from build123d import *

# Parameters (mm, degrees)
F1_DEPTH    = 924
F2_T1_DEPTH = 1877.7738168108


# Not quite as in the source:
# - a fillet or chamfer that OpenCascade refuses, or shapes differently, is made with other operations: its cross-section is extruded or revolved along the edge and cut away or added


with BuildPart() as f1:
    # F0 (on Right) → F1 (new body, symmetric)
    with BuildSketch(Plane.YZ):
        with BuildLine():
            ThreePointArc((-20.915, -48.8), (-20.3292135624, -50.2142135624), (-18.915, -50.8))
            Line((-18.915, -50.8), (18.915, -50.8))
            ThreePointArc((18.915, -50.8), (20.3292135624, -50.2142135624), (20.915, -48.8))
            Line((20.915, -48.8), (20.915, 48.8))
            ThreePointArc((20.915, 48.8), (20.3292135624, 50.2142135624), (18.915, 50.8))
            Line((18.915, 50.8), (-18.915, 50.8))
            ThreePointArc((-18.915, 50.8), (-20.3292135624, 50.2142135624), (-20.915, 48.8))
            Line((-20.915, 48.8), (-20.915, 44.8355484375))
            Line((-20.915, 44.8355484375), (10.0807787137, 42.1237691829))
            ThreePointArc((10.0807787137, 42.1237691829), (13.3313866841, 40.5207467305), (14.645, 37.1427956924))
            Line((14.645, 37.1427956924), (14.645, -37.1427956924))
            ThreePointArc((14.645, -37.1427956924), (13.3313866841, -40.5207467305), (10.0807787137, -42.1237691829))
            Line((10.0807787137, -42.1237691829), (-20.915, -44.8355484375))
            Line((-20.915, -44.8355484375), (-20.915, -48.8))
        make_face()
    extrude(amount=F1_DEPTH, both=True)

    # F2: fillet of radius 7 on 2 edges, made by hand

    # F2_s2 → F2_t1 (cut)
    with BuildSketch(Plane.YZ.offset(-938.8869084054)):
        with BuildLine():
            ThreePointArc((-20.915, -48.8), (-18.5934823683, -45.7054865005), (-14.9828963102, -44.3165566138))
            Line((-14.9828963102, -44.3165566138), (-14.9950981142, -44.177089356))
            Line((-14.9950981142, -44.177089356), (-20.927201804, -44.6960811798))
            Line((-20.927201804, -44.6960811798), (-21.055, -44.8355484375))
            ThreePointArc((-21.055, -44.8355484375), (-21.055, -46.8177742187), (-21.0458438778, -48.75020161))
            Line((-21.0458438778, -48.75020161), (-20.915, -48.8))
        make_face()
        with BuildLine():
            ThreePointArc((-14.9828963102, 44.3165566138), (-18.5934823683, 45.7054865005), (-20.915, 48.8))
            Line((-20.915, 48.8), (-21.0458438778, 48.75020161))
            ThreePointArc((-21.0458438778, 48.75020161), (-21.055, 46.8177742187), (-21.055, 44.8355484375))
            Line((-21.055, 44.8355484375), (-20.927201804, 44.6960811798))
            Line((-20.927201804, 44.6960811798), (-14.9950981142, 44.177089356))
            Line((-14.9950981142, 44.177089356), (-14.9828963102, 44.3165566138))
        make_face()
    extrude(amount=F2_T1_DEPTH, mode=Mode.SUBTRACT)


solid = f1.part
For this review, take the finished solid that the model builds, in its own axes (mm). A direction names the side the tool comes from. Round coordinates to 2 decimals unless told otherwise and drop trailing zeros. Loops run counter-clockwise (first coordinate to the right, second up) from the corner with the lowest first, then second, coordinate; pieces in that order, holes last. Notation, with made-up numbers: (33, 37.5) - (79, 37.5) arc R21 cw to (79, 44.5) - close; hole circle Ø4 at (3, -15.5). An arc over 180 degrees is marked (long way). Use one line per item in the form item = value.
Item 1: Consider section C-C on z = -1. Write out the cut boundary in (x, y) (3 decimals), then the cut area to 3 significant figures.
Answers:
outline = (-924, 14.645) - (924, 14.645) - (924, 20.915) - (-924, 20.915) - close
area = 11,600 mm^2
Item 2: Consider section A-A on x = -666. Write out the cut boundary in (y, z) (3 decimals).
Answers:
outline = (-20.915, -48.8) arc R2 ccw to (-18.915, -50.8) - (18.915, -50.8) arc R2 ccw to (20.915, -48.8) - (20.915, 48.8) arc R2 ccw to (18.915, 50.8) - (-18.915, 50.8) arc R2 ccw to (-20.915, 48.8) arc R7 ccw to (-14.983, 44.317) - (10.081, 42.124) arc R5 cw to (14.645, 37.143) - (14.645, -37.143) arc R5 cw to (10.081, -42.124) - (-14.983, -44.317) arc R7 ccw to start
Item 3: Clearance check with flat-ended pins moving along their axes: P1, Ø4, axis at x = -621.5, z = -20.5, coming from the -Y side (3 decimals); P2, Ø8, axis at x = -631, z = 37, coming from the -Y side. State where each tip first meets the part, or that it passes through.
Answers:
P1 = 14.645
P2 = 12.83
Item 4: Tool access review of faces 1 (the flat face through (13, 14.645, 1)), 2 (the flat face through (-924, 15, 0)): name each direction out of +Z, -Z, +X, -X, +Y, -Y from which nothing blocks a thin tool from reaching the whole face with its end or side.
Answers:
face_1 = +X, -X, -Y
face_2 = +Z, -Z, -X, +Y, -Y
Item 5: Consider section B-B on y = -4.5. Write out the cut boundary in (x, z), then the cut area to 3 significant figures.
Answers:
outline = (-924, -50.8) - (924, -50.8) - (924, -43.4) - (-924, -43.4) - close; (-924, 43.4) - (924, 43.4) - (924, 50.8) - (-924, 50.8) - close
area = 27,400 mm^2
Item 6: For line 1 (Z direction, x = 154, y = -13); line 2 (Z direction, x = -211, y = 7); line 3 (Y direction, x = -36.5, z = -37.5) (3 decimals), list the stretches that pass through material, from the lowest coordinate up.
Answers:
line_1 = -50.8 to -44.14, 44.14 to 50.8
line_2 = -50.8 to -42.39, 42.39 to 50.8
line_3 = 14.632 to 20.915
